Can you work these out from the drawing? Everything is in mm from the part's minimum corner. Give positions to 0.01 mm unless a question says otherwise; leave off trailing zeros. Order: outer loops, then holes, each group sorted by start corner. A loop starts at its lowest first (then second) coordinate and runs counter-clockwise, first axis right, second up. Notation, with made-up numbers: (37.25, 6.5) - (94.25, 6.5) arc R29 ccw to (94.25, 40.5) - close; hole circle Ø10 at (67.25, 47). An arc over 180 degrees is marked (long way). Answer as a JSON object with one key per item and string values.
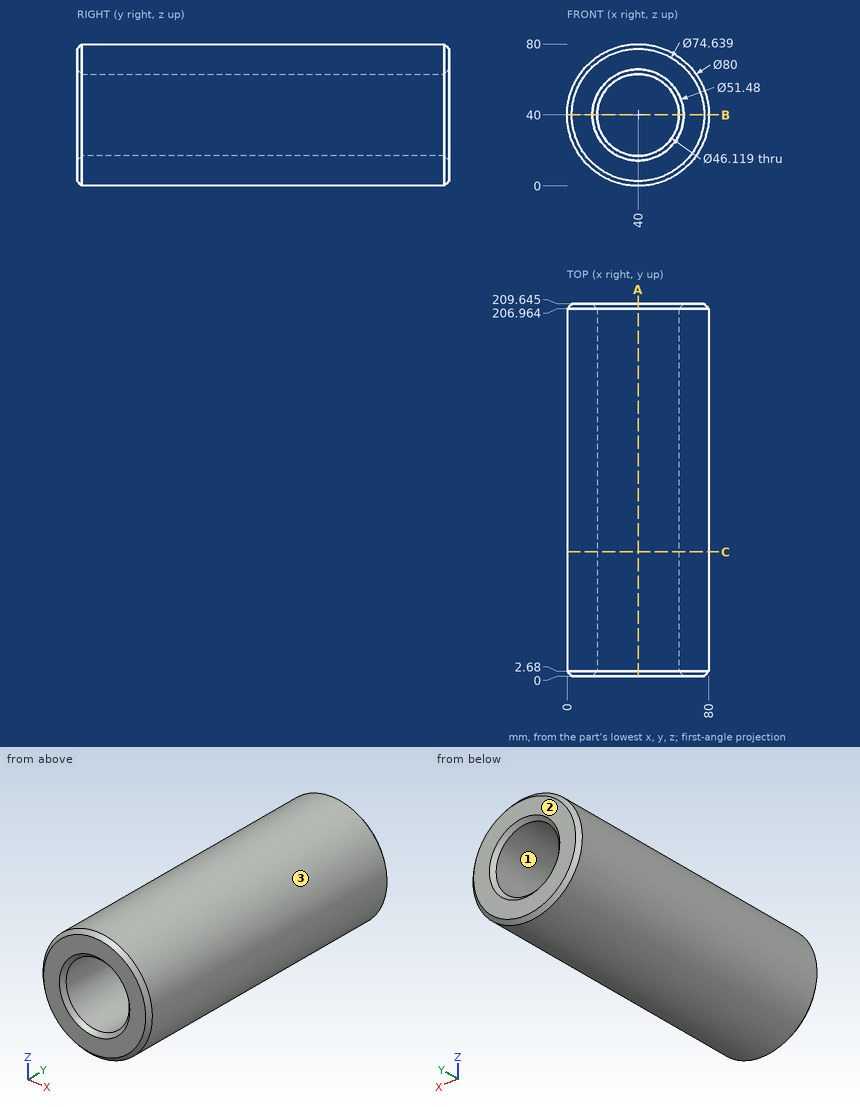
Q1. If we section it at A-A, the plane x = 40: Please give me the cut outline in (y, z) (1 decimal), then the cut area to 3 significant figures.
Recorded:
{"outline": "(0, 2.7) - (2.7, 0) - (207, 0) - (209.6, 2.7) - (209.6, 14.3) - (207, 16.9) - (2.7, 16.9) - (0, 14.3) - close; (0, 65.7) - (2.7, 63.1) - (207, 63.1) - (209.6, 65.7) - (209.6, 77.3) - (207, 80) - (2.7, 80) - (0, 77.3) - close", "area": "7,070 mm^2"}
Q2. We'd pull the mould along X, two halves only. Please class the marked faces 1, 2 and 3: released by +X, released by -X, zero draft, split by the parting line, or undercut.
Recorded:
{"face 1": "undercut", "face 2": "zero draft", "face 3": "split by the parting line"}
Q3. If we section it at C-C, the plane y = 70: Please give me the cut outline in (x, z).
Recorded:
{"outline": "circle Ø80 at (40, 40); hole circle Ø46.12 at (40, 40)"}
Q4. I need wall thicknesses on L1, parallel to X at y = 166, z = 40; L2, parallel to Z at x = 50, y = 18; L3, parallel to Z at x = 22, y = 103 (1 decimal). Which ranges of each line are inside material? Lowest first, please.
Recorded:
{"L1": "x = 0 to 16.94, 63.06 to 80", "L2": "z = 1.27 to 19.22, 60.78 to 78.73", "L3": "z = 4.3 to 25.6, 54.4 to 75.7"}
Q5. If we section it at B-B, the plane z = 40: Please give me the cut outline in (x, y) (1 decimal), then the cut area to 3 significant figures.
Recorded:
{"outline": "(0, 2.7) - (2.7, 0) - (14.3, 0) - (16.9, 2.7) - (16.9, 207) - (14.3, 209.6) - (2.7, 209.6) - (0, 207) - close; (63.1, 2.7) - (65.7, 0) - (77.3, 0) - (80, 2.7) - (80, 207) - (77.3, 209.6) - (65.7, 209.6) - (63.1, 207) - close", "area": "7,070 mm^2"}
Q6. I'm going to push flat-ended pins straight in: pin 1 Ø5 at (y, z) = (35.5, 62.5) entering from +X; pin 2 Ø1.5 at (x, y) = (35, 125) entering from +Z; pin 3 Ø3 at (y, z) = (69, 38.5) entering from +X. Where does each tip first touch, or does it pass through?
Recorded:
{"pin 1": "stops at x = 74.64", "pin 2": "stops at z = 79.77", "pin 3": "stops at x = 80"}
